Work out the finished part from the listing and answer in its coordinate system (mm). A direction names the side the tool comes from. Round coordinates to 2 decimals unless told otherwise and drop trailing zeros. Write each loop counter-clockwise with the first axis right and the second up, starting at its lowest first coordinate (ties: lowest second). Pieces come first, ordered by that corner, then holes. Notation, with made-up numbers: M 49.5,17.25 L 56.5,17.25 A19 cw 56.5,44.25 Z; hole C 66,-25.5 d2. An arc over 180 degrees is marked long. One line per item, written item: value. Start each with the question number.
Q1. Given pin 1 Ø5.5 at (y, z) = (20, -11.5) entering from +X; pin 2 Ø20 at (x, y) = (44, 15.5) entering from +Z, each flat-ended and moving along its own axis, determine where each tip first touches the part or whether it passes through.
Q2. Find section A-A (y = 12.5). Write down the section's boundary in (x, z), and give its area (3 significant figures).
Q3. Consider probe 1 along Y at (x, z) = (103.5, -10); probe 2 along X at (y, z) = (22.5, -17.5); probe 3 along X at (y, z) = (17, -6). Determine where each line is inside the solid, lowest interval first.
Q4. A tool of negligible diameter and unlimited length cuts with its end or side. For faces 5 (the flat face through (62, 0, -10)), 6 (the cylindrical face through (105.916, 24.638, -12.957)), 7 (the flat face through (49, 20, -13)), 8 (the flat face through (97, 20, 0)), 9 (the flat face through (94, 20, -3)), from which of +Z, -Z, +X, -X, +Y, -Y can it reach the whole face along a straight path? Write none if from no direction.
Q5. Find section C-C (z = -10). Write down the section's boundary in (x, y), and give its area (3 significant figures).
Q6. Find section D-D (x = 34.5). Write down the section's boundary in (y, z), and give its area (3 significant figures).
Q7. Find section B-B (z = -3). Write down the section's boundary in (x, y).
Q8. The mould has two halves that part along Z. Classify faces 1 (the flat face through (100, 20, -10)), 2 (the cylindrical face through (105.92, 11.7, -8.16)), 3 (the flat face through (0, 20, -10)), 4 (the flat face through (97, 20, -20)): released by +Z, released by -Z, zero draft, split by the parting line, or undercut.
from build123d import *

# Parameters (mm, degrees)
BOSS_EXTRUDE2_DEPTH = 40
SKETCH2_R           = 8.5
SKETCH2_R_2         = 5.5
BOSS_EXTRUDE3_DEPTH = 12


with BuildPart() as part:
    # Sketch1 → Boss-Extrude2 (new body)
    with BuildSketch(Plane(origin=(0, 0, 0), x_dir=(1, 0, 0), z_dir=(0, 1, 0))):
        Polygon((0, 0), (0, 20), (6, 20), (6, 13), (94, 13), (94, 20), (100, 20), (100, 0), (94, 0), (94, 7), (6, 7), (6, 0), align=None)
    extrude(amount=BOSS_EXTRUDE2_DEPTH)

    # Sketch2 → Boss-Extrude3 (add)
    with BuildSketch(Plane(origin=(100, 0, 0), x_dir=(0, 0, -1), z_dir=(1, 0, 0))):
        with Locations((10, 20)):
            Circle(SKETCH2_R)
        with Locations((10, 20)):
            Circle(SKETCH2_R_2, mode=Mode.SUBTRACT)
    extrude(amount=BOSS_EXTRUDE3_DEPTH)


solid = part.part
The answers:
1. pin 1: x = 100
1. pin 2: z = -7
2. outline: M 0,-20 L 6,-20 L 6,-13 L 94,-13 L 94,-20 L 100,-20 L 100,-14 L 112,-14 L 112,-6 L 100,-6 L 100,0 L 94,0 L 94,-7 L 6,-7 L 6,0 L 0,0 Z
2. area: 864 mm2
3. probe 1: 11.5 to 14.5, 25.5 to 28.5
3. probe 2: 0 to 6, 94 to 112
3. probe 3: 0 to 6, 94 to 100
4. face 5: +Z, -Z, +X, -X, -Y
4. face 6: +X
4. face 7: -Z, +Y, -Y
4. face 8: +Z, +X, -X, +Y, -Y
4. face 9: +Z, +Y, -Y
5. outline: M 0,0 L 100,0 L 100,11.5 L 112,11.5 L 112,14.5 L 100,14.5 L 100,25.5 L 112,25.5 L 112,28.5 L 100,28.5 L 100,40 L 0,40 Z
5. area: 4,070 mm2
6. outline: M 0,-13 L 40,-13 L 40,-7 L 0,-7 Z
6. area: 240 mm2
7. outline: M 0,0 L 6,0 L 6,40 L 0,40 Z; M 94,0 L 100,0 L 100,15.18 L 112,15.18 L 112,24.82 L 100,24.82 L 100,40 L 94,40 Z
8. face 1: undercut
8. face 2: split by the parting line
8. face 3: zero draft
8. face 4: released by -Z
